Geometry: final body of the model. Coordinates: model frame, mm. Face numbers are marked on the shaded views. A direction names the side the tool comes from. Give positions to 0.01 mm unless a question says otherwise; leave off trailing zeros. Write each loop counter-clockwise with the first axis right and the second up, starting at its lowest first coordinate (ties: lowest second). Pieces come first, ordered by that corner, then holes. Notation, with made-up numbers: M 45.5,18.5 L 55.5,18.5 A22 ccw 55.5,54.5 Z; hole C 28,14.25 d3. An arc over 180 degrees is marked long. Answer as a JSON object with one key per item and string values.
from build123d import *

# Parameters (mm, degrees)
F0_W     = 20
F0_H     = 2.8
F1_DEPTH = 16
F2_R     = 10
F3_R     = 5


with BuildPart() as f1:
    # F0 (on Front) → F1 (new body)
    with BuildSketch(Plane.XZ):
        Polygon((-30, 0), (0, 0), (0, 2.8), (-10, 2.8), (-30, 2.8), align=None)
        with Locations((10, 1.4)):
            Rectangle(F0_W, F0_H)
        Polygon((-10, 2.8), (0, 2.8), (0, 55), (10, 55), (10, 57.8), (-10, 57.8), align=None)
    extrude(amount=F1_DEPTH)

    # F2
    f2_edges = [f1.edges().sort_by_distance(p)[0] for p in [
        (-10, -8, 2.8),
        (0, -8, 2.8),
    ]]
    fillet(f2_edges, radius=F2_R)

    # F3
    f3_edges = [f1.edges().sort_by_distance(p)[0] for p in [
        (-10, -8, 57.8),
        (0, -8, 55),
    ]]
    fillet(f3_edges, radius=F3_R)


solid = f1.part
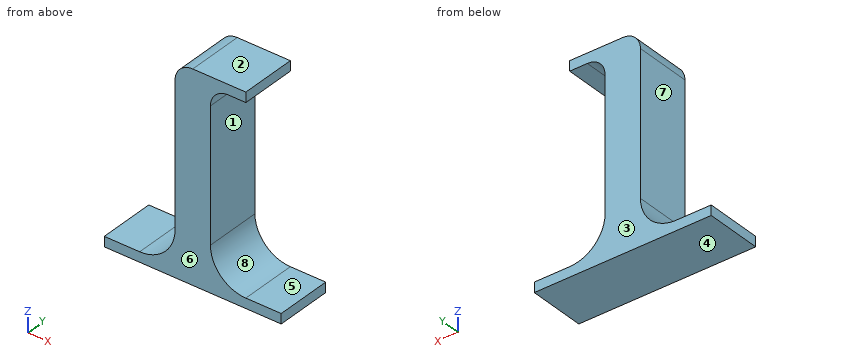
1) Pull-direction query (Z, two-part tool) for the marked faces 1, 2, 3 and 4; classes: pulls with the +Z half, pulls with the -Z half, needs draft (parallel to the pull), parting line crosses it, or undercut.
Geometry check:
{"face 1": "undercut", "face 2": "pulls with the +Z half", "face 3": "needs draft", "face 4": "pulls with the -Z half"}
2) Set-up query: the marked faces 5, 6, 7 and 8. Return all of +Z, -Z, +X, -X, +Y, -Y with unobstructed straight access to the full face (end or side cutting, diameter ignored); none if empty.
Geometry check:
{"face 5": "+Z, +X, +Y, -Y", "face 6": "+Z, -Z, +X, -X, -Y", "face 7": "+Z, -X, +Y, -Y", "face 8": "+X, +Y, -Y"}
3) Cut plane B-B on x = 2.5. Return loops of the section in (y, z), and give its area (3 significant figures).
Geometry check:
{"outline": "M -16,0 L 0,0 L 0,6.19 L -16,6.19 Z; M -16,54.33 L 0,54.33 L 0,57.8 L -16,57.8 Z", "area": "154 mm2"}
4) Cut plane A-A on y = -2. Return loops of the section in (x, z), and give its area (3 significant figures).
Geometry check:
{"outline": "M -30,0 L 20,0 L 20,2.8 L 10,2.8 A10 cw 0,12.8 L 0,50 A5 cw 5,55 L 10,55 L 10,57.8 L -5,57.8 A5 ccw -10,52.8 L -10,12.8 A10 cw -20,2.8 L -30,2.8 Z", "area": "761 mm2"}
5) Contact query for flat-ended pins moving along their axis: P1, Ø4, axis at y = -13, z = 40.5, coming from the +X side; P2, Ø5, axis at y = -9.5, z = 43.5, coming from the -X side; P3, Ø1.4, axis at y = -11.5, z = 56.5, coming from the +X side; P4, Ø6, axis at x = 6, z = 50.5, coming from the +Y side. Output: stop coordinate, or through.
Geometry check:
{"P1": "stops at x = 0", "P2": "stops at x = -10", "P3": "stops at x = 10", "P4": "passes through"}
6) Cut plane C-C on z = 44.5. Return loops of the section in (x, y), and give its area (3 significant figures).
Geometry check:
{"outline": "M -10,-16 L 0,-16 L 0,0 L -10,0 Z", "area": "160 mm2"}
7) Line query: line 1 (X direction, y = -10.25, z = 45); line 2 (Z direction, x = -25, y = -9.5); line 3 (X direction, y = -0.75, z = 10.5). Output: solid intervals per line, ascending. Write a range as from..to.
Geometry check:
{"line 1": "x = -10..0", "line 2": "z = 0..2.8", "line 3": "x = -10.27..0.27"}
8) Cut plane D-D on x = 8.5. Return loops of the section in (y, z).
Geometry check:
{"outline": "M -16,0 L 0,0 L 0,2.91 L -16,2.91 Z; M -16,55 L 0,55 L 0,57.8 L -16,57.8 Z"}
